The listing builds one solid part. Answer for the finished solid, in the listing's coordinates (mm). A direction names the side the tool comes from. Give positions to 0.01 mm unless a question says otherwise; leave off trailing zeros. Loops run counter-clockwise (first coordinate to the right, second up) from the corner with the lowest first, then second, coordinate; pieces in that order, holes last. Notation, with made-up numbers: (29.25, -30) - (69.25, -30) arc R20 ccw to (69.25, 3) - close; hole circle Ø10 at (0, 87). An arc over 180 degrees is marked (long way). Write each question's results on one line, items separated by ' | '.
from build123d import *

# Parameters (mm, degrees)
SKETCH1_R           = 20
SKETCH1_R_2         = 3.25
BOSS_EXTRUDE1_DEPTH = 12
SKETCH2_R           = 6.45
CUT_EXTRUDE1_DEPTH  = 8
SKETCH3_R           = 3
CUT_EXTRUDE2_DEPTH  = 31.724582991
CIRPATTERN1_COUNT   = 10


with BuildPart() as part:
    # Sketch1 → Boss-Extrude1 (new body)
    with BuildSketch(Plane(origin=(0, 0, 0), x_dir=(1, 0, 0), z_dir=(0, 1, 0))):
        with Locations(Location((0, 0, 0), (0, 0, 270))):
            Circle(SKETCH1_R)
        with Locations(Location((0, 0, 0), (0, 0, 270))):
            Circle(SKETCH1_R_2, mode=Mode.SUBTRACT)
    extrude(amount=BOSS_EXTRUDE1_DEPTH)

    # Sketch2 → Cut-Extrude1 (cut)
    with BuildSketch(Plane(origin=(0, 12, 0), x_dir=(1, 0, 0), z_dir=(0, 1, 0))):
        with Locations(Location((0, 0, 0), (0, 0, 270))):
            Circle(SKETCH2_R)
    extrude(amount=-CUT_EXTRUDE1_DEPTH, mode=Mode.SUBTRACT)

    # Sketch3 → Cut-Extrude2 (cut, through all)
    with BuildSketch(Plane(origin=(0, 12, 0), x_dir=(1, 0, 0), z_dir=(0, 1, 0))):
        with Locations((20, 0)):
            Circle(SKETCH3_R)
    cut_extrude2 = extrude(amount=-CUT_EXTRUDE2_DEPTH, mode=Mode.SUBTRACT)

    # CirPattern1: Cut-Extrude2 ×10 about axis
    cirpattern1_axis = Axis((0, 0, 0), (0, 1, 0))
    for i in range(1, CIRPATTERN1_COUNT):
        add(cut_extrude2.rotate(cirpattern1_axis, i * 360 / CIRPATTERN1_COUNT), mode=Mode.SUBTRACT)


solid = part.part
Item 1: For faces 5 (the face through (2, 4, -3)), 6 (the face through (0, 6, 20)), determine the directions among +Z, -Z, +X, -X, +Y, -Y from which every point of the face is accessible in a straight line to the end or side of a thin tool.
Values found:
face 5: +Y | face 6: +Z, +Y, -Y
Item 2: For a pull along X with two mould halves and no side action, classify faces 1 (the face through (-13.72, 6.08, 10.04)), 2 (the face through (17, 6, 0)), 3 (the face through (-17, 6, 0)), 4 (the face through (-1.978, 1.972, -2.579)) as released by +X, released by -X, zero draft, split by the parting line, or undercut.
Values found:
face 1: undercut | face 2: released by +X | face 3: released by -X | face 4: undercut
Item 3: Find the intervals of material crossed by line 1 along Z through (x, y) = (0, 1.95); line 2 along X through (y, z) = (1, 16.5); line 3 along X through (y, z) = (4, 9), in increasing order. Write a range as [from, to].
Values found:
line 1: z = [-20, -3.25], [3.25, 20] | line 2: x = [-11.3, -7.81], [-4.55, 4.55], [7.81, 11.3] | line 3: x = [-17.86, -17.37], [-14.99, 14.99], [17.37, 17.86]
Item 4: A cutting plane is placed at C-C, the plane x = 0. Determine the outline of the cut face in (y, z).
Values found:
outline: (0, -20) - (12, -20) - (12, -6.45) - (4, -6.45) - (4, -3.25) - (0, -3.25) - close; (0, 3.25) - (4, 3.25) - (4, 6.45) - (12, 6.45) - (12, 20) - (0, 20) - close
Item 5: A cutting plane is placed at B-B, the plane z = 0. Determine the outline of the cut face in (x, y), plus the area to 3 significant figures.
Values found:
outline: (-17, 0) - (-3.25, 0) - (-3.25, 4) - (-6.45, 4) - (-6.45, 12) - (-17, 12) - close; (3.25, 0) - (17, 0) - (17, 12) - (6.45, 12) - (6.45, 4) - (3.25, 4) - close | area: 279 mm²
Item 6: Flat-ended cylindrical pins translate along their axes: P1, Ø1, axis at y = 6, z = -15, coming from the -X side (3 decimals); P2, Ø10.5, axis at x = 0, z = 0, coming from the +Y side; P3, Ø1, axis at y = 3.5, z = 9.5, coming from the -X side. Find the tip coordinate at first contact, or state that the pin passes through.
Values found:
P1: stops at x = -13.775 | P2: stops at y = 4 | P3: stops at x = -17.86
Item 7: A cutting plane is placed at D-D, the plane x = -4. Determine the outline of the cut face in (y, z), plus the area to 3 significant figures.
Values found:
outline: (0, -16.96) - (12, -16.96) - (12, -5.06) - (4, -5.06) - (4, 5.06) - (12, 5.06) - (12, 16.96) - (0, 16.96) - close | area: 326 mm²
Item 8: A cutting plane is placed at A-A, the plane y = 3.25. Determine the outline of the cut face in (x, z) (3 decimals), plus the area to 3 significant figures.
Values found:
outline: (-19.775, -2.992) arc R20 ccw to (-17.757, -9.203) arc R3 cw to (-14.24, -14.044) arc R20 ccw to (-8.956, -17.883) arc R3 cw to (-3.266, -19.732) arc R20 ccw to (3.266, -19.732) arc R3 cw to (8.956, -17.883) arc R20 ccw to (14.24, -14.044) arc R3 cw to (17.757, -9.203) arc R20 ccw to (19.775, -2.992) arc R3 cw to (19.775, 2.992) arc R20 ccw to (17.757, 9.203) arc R3 cw to (14.24, 14.044) arc R20 ccw to (8.956, 17.883) arc R3 cw to (3.266, 19.732) arc R20 ccw to (-3.266, 19.732) arc R3 cw to (-8.956, 17.883) arc R20 ccw to (-14.24, 14.044) arc R3 cw to (-17.757, 9.203) arc R20 ccw to (-19.775, 2.992) arc R3 cw to start; hole circle Ø6.5 at (0, 0) | area: 1,090 mm²
